Verification items for the finished model (mm, model axes). Round coordinates to 2 decimals unless told otherwise and drop trailing zeros. Write each loop counter-clockwise with the first axis right and the second up, starting at its lowest first coordinate (ties: lowest second). Pieces come first, ordered by that corner, then holes. Notation, with made-up numbers: M 76.5,-27 L 135.5,-27 A9 cw 135.5,-17 Z; hole C 58,43 d11. An arc over 180 degrees is marked long. Write each question's results on one line, items separated by ' | '.
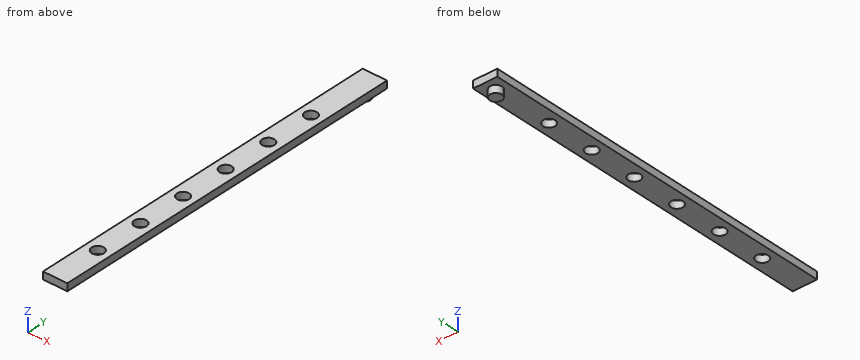
from build123d import *

# Parameters (mm, degrees)
SKETCH_1_W      = 10
SKETCH_1_H      = 150
SKETCH_1_R      = 2.5
EXTRUDE_1_DEPTH = 3
SKETCH_2_R      = 2.5
EXTRUDE_2_DEPTH = 6


with BuildPart() as part:
    # 草圖1 → 填料-伸長1 (new body)
    with BuildSketch(Plane.XY):
        Rectangle(SKETCH_1_W, SKETCH_1_H)
        with Locations((0, -55)):
            Circle(SKETCH_1_R, mode=Mode.SUBTRACT)
        with Locations((0, -35)):
            Circle(SKETCH_1_R, mode=Mode.SUBTRACT)
        with Locations((0, -15)):
            Circle(SKETCH_1_R, mode=Mode.SUBTRACT)
        with Locations((0, 5)):
            Circle(SKETCH_1_R, mode=Mode.SUBTRACT)
        with Locations((0, 25)):
            Circle(SKETCH_1_R, mode=Mode.SUBTRACT)
        with Locations((0, 45)):
            Circle(SKETCH_1_R, mode=Mode.SUBTRACT)
    extrude(amount=EXTRUDE_1_DEPTH)

    # 草圖2 → 填料-伸長2 (add)
    with BuildSketch(Plane.XY.offset(3)):
        with Locations((0, 70)):
            Circle(SKETCH_2_R)
    extrude(amount=-EXTRUDE_2_DEPTH)


solid = part.part
1) Material ranges on line 1 (Z direction, x = 1.5, y = 52.5); line 2 (Y direction, x = 0.5, z = -1.9), recorded low to high. Write a range as [from, to].
Calculated:
line 1: z = [0, 3] | line 2: y = [67.55, 72.45]
2) Sectioned sample at B-B, the plane y = 45. Record the cut outline in (x, z), and give its area (3 significant figures).
Calculated:
outline: M -5,0 L -2.5,0 L -2.5,3 L -5,3 Z; M 2.5,0 L 5,0 L 5,3 L 2.5,3 Z | area: 15.0 mm²
3) Sectioned sample at A-A, the plane x = 0. Count the separate pieces of the cut face and the enclosed holes in it, and give its area (3 significant figures).
Calculated:
separate pieces: 7 | enclosed holes: 0 | area: 375 mm²
4) Sectioned sample at C-C, the plane z = 1.75. Record the cut outline in (x, y).
Calculated:
outline: M -5,-75 L 5,-75 L 5,75 L -5,75 Z; hole C 0,-55 d5; hole C 0,-35 d5; hole C 0,-15 d5; hole C 0,5 d5; hole C 0,25 d5; hole C 0,45 d5
5) Sectioned sample at D-D, the plane y = 70. Record the cut outline in (x, z).
Calculated:
outline: M -5,0 L -2.5,0 L -2.5,-3 L 2.5,-3 L 2.5,0 L 5,0 L 5,3 L -5,3 Z
6) Depth check by flat-ended pin: P1, Ø3, axis at x = 0, y = -55, coming from the +Z side; P2, Ø3, axis at x = -1.5, y = 52, coming from the -Z side. Enter the tip coordinate at first touch or a pass-through.
Calculated:
P1: passes through | P2: stops at z = 0
